Source: CAD feature listing. Evaluate the final solid. Frame: model axes, mm. A direction names the side the tool comes from. Round coordinates to 2 decimals unless told otherwise and drop trailing zeros. Order: outer loops, then holes, each group sorted by start corner. A loop starts at its lowest first (then second) coordinate and runs counter-clockwise, first axis right, second up. Notation, with made-up numbers: (73, 49) -> (120, 49) arc R6 cw to (120, 53) -> close; hole circle Ø11 at (-33.5, 19). An arc over 180 degrees is marked (long way). Answer as CSV lines item,"result".
Autodesk Inventor part; units mm, degrees
ref_plane "YZ Plane" through (0, 0, 0) normal (1, 0, 0) x (0, 1, 0)
ref_plane "XZ Plane" through (0, 0, 0) normal (0, 1, 0) x (-1, 0, 0)
ref_plane "XY Plane" through (0, 0, 0) normal (0, 0, 1) x (1, 0, 0)
sketch "Sketch1" plane through (0, 0, 0) normal (0, 1, 0) x (-1, 0, 0)
  circle A0 centre (0, 0) radius 21
  circle A1 centre (0, 25) radius 2.5
  circle A2 centre (0, -25) radius 2.5
  line L0 (-31, 54) -> (-19, 54)
  line L1 (-19, 54) -> (-19, 30)
  line L2 (-19, 30) -> (-31, 30)
  line L3 (-31, 30) -> (-31, 54)
  line L4 (19, 54) -> (31, 54)
  line L5 (31, 54) -> (31, 30)
  line L6 (31, 30) -> (19, 30)
  line L7 (19, 30) -> (19, 54)
  line L8 (-31, -30) -> (-19, -30)
  line L9 (-19, -30) -> (-19, -54)
  line L10 (-19, -54) -> (-31, -54)
  line L11 (-31, -54) -> (-31, -30)
  line L12 (19, -30) -> (31, -30)
  line L13 (31, -30) -> (31, -54)
  line L14 (31, -54) -> (19, -54)
  line L15 (19, -54) -> (19, -30)
  line L16 (-36, 59) -> (36, 59)
  line L17 (36, 59) -> (36, -59)
  line L18 (36, -59) -> (-36, -59)
  line L19 (-36, -59) -> (-36, 59)
  dimension "d2" = 5
  dimension "d4" = 5
  dimension "d9" = 12
  dimension "d10" = 24
  dimension "d11" = 12
  dimension "d12" = 24
  dimension "d13" = 12
  dimension "d14" = 24
  dimension "d15" = 12
  dimension "d16" = 24
extrude "Extrusion1" add sketch "Sketch1" along normal blind 5
properties part number "X_Carriage_V1" material "Ash"
1. Section query A-A on z = 46. Return loops of the section in (x, y), and give its area (3 significant figures).
Results below:
outline,"(-36, 0) -> (-31, 0) -> (-31, 5) -> (-36, 5) -> close; (-19, 0) -> (19, 0) -> (19, 5) -> (-19, 5) -> close; (31, 0) -> (36, 0) -> (36, 5) -> (31, 5) -> close"
area,"240 mm2"
2. Mould query, pull axis Z, two halves, no side actions, for faces 1 (the flat face through (17, 5, 14)), 2 (the flat face through (1, 2, 59)), 3 (the flat face through (-25, 2, 54)). Classes: released by +Z, released by -Z, zero draft, split by the parting line, or undercut.
Results below:
face 1,"zero draft"
face 2,"released by +Z"
face 3,"undercut"
3. Section query D-D on z = 0. Return loops of the section in (x, y).
Results below:
outline,"(-36, 0) -> (-21, 0) -> (-21, 5) -> (-36, 5) -> close; (21, 0) -> (36, 0) -> (36, 5) -> (21, 5) -> close"
4. Section query C-C on y = 1.95. Return loops of the section in (x, z), and give its area (3 significant figures).
Results below:
outline,"(-36, -59) -> (36, -59) -> (36, 59) -> (-36, 59) -> close; hole (-31, -54) -> (-19, -54) -> (-19, -30) -> (-31, -30) -> close; hole (-31, 30) -> (-19, 30) -> (-19, 54) -> (-31, 54) -> close; hole circle Ø42 at (0, 0); hole circle Ø5 at (0, -25); hole circle Ø5 at (0, 25); hole (19, -54) -> (31, -54) -> (31, -30) -> (19, -30) -> close; hole (19, 30) -> (31, 30) -> (31, 54) -> (19, 54) -> close"
area,"5,920 mm2"
5. Line query: L1, parallel to Z at x = 24, y = 4.7; L2, parallel to X at y = 3.3, z = -49.5; L3, parallel to Z at x = 0, y = 3.05. Output: solid intervals per line, ascending. Write a range as [from, to].
Results below:
L1,"[-59, -54], [-30, 30], [54, 59]"
L2,"[-36, -31], [-19, 19], [31, 36]"
L3,"[-59, -27.5], [-22.5, -21], [21, 22.5], [27.5, 59]"
6. Reachability of faces 4 (the flat face through (17, 0, 14)), 5 (the flat face through (25, 2, -30)) from +Z, -Z, +X, -X, +Y, -Y: full face, straight path, thin tool, end or side. Return the list, or none.
Results below:
face 4,"+Z, -Z, +X, -X, -Y"
face 5,"+Y, -Y"
7. Section query B-B on x = -23.5. Return loops of the section in (y, z), and give its area (3 significant figures).
Results below:
outline,"(0, -59) -> (5, -59) -> (5, -54) -> (0, -54) -> close; (0, -30) -> (5, -30) -> (5, 30) -> (0, 30) -> close; (0, 54) -> (5, 54) -> (5, 59) -> (0, 59) -> close"
area,"350 mm2"
